Check sheet for the modelled part. Datum: model origin and axes. Units: mm. A direction names the side the tool comes from. Give positions to 0.01 mm unless a question says otherwise; leave off trailing zeros. Write each loop counter-clockwise with the first axis right and the second up, starting at its lowest first coordinate (ties: lowest second). Pieces come first, ordered by that corner, then holes.
from build123d import *
from OCP.BRepFilletAPI import BRepFilletAPI_MakeChamfer

# Parameters (mm, degrees)
SKETCH1_W           = 20.32
SKETCH1_H           = 40.64
BOSS_EXTRUDE1_DEPTH = 25.4
SKETCH2_W           = 20.32
SKETCH2_H           = 40.64
BOSS_EXTRUDE2_DEPTH = 2.38
SKETCH3_W           = 20.32
SKETCH3_H           = 40.5892
BOSS_EXTRUDE3_DEPTH = 4.445
BOSS_EXTRUDE4_DEPTH = 2.38
SKETCH6_R           = 7.62
BOSS_EXTRUDE5_DEPTH = 3.495
CHAMFER1_SIZE       = 2.54
CHAMFER1_SIZE2      = 1.466469684
BOSS_EXTRUDE6_DEPTH = 0.635
SKETCH9_R           = 2.78
BOSS_EXTRUDE7_DEPTH = 7
CHAMFER2_SIZE       = 2.54
CHAMFER2_SIZE2      = 1.466469684
FILLET1_R           = 1
FILLET2_R           = 1.5
SKETCH10_W          = 6.35
SKETCH10_H          = 2.54
SKETCH10_W_2        = 5.08
SKETCH10_H_2        = 1.27
BOSS_EXTRUDE8_DEPTH = 2.4


with BuildPart() as part:
    # Sketch1 → Boss-Extrude1 (new body)
    with BuildSketch(Plane(origin=(0, 0, 0), x_dir=(1, 0, 0), z_dir=(0, 1, 0))):
        with Locations((0, -10.16)):
            Rectangle(SKETCH1_W, SKETCH1_H)
    extrude(amount=BOSS_EXTRUDE1_DEPTH)

    # Sketch2 → Boss-Extrude2 (add)
    with BuildSketch(Plane(origin=(0, 25.4, 0), x_dir=(1, 0, 0), z_dir=(0, 1, 0))):
        with BuildLine():
            ThreePointArc((-5.58, 15.384213562), (-5.08, 12.47), (-4.58, 15.384213562))
            Line((-4.58, 15.384213562), (-4.58, 16.4846))
            Line((-4.58, 16.4846), (4.58, 16.4846))
            Line((4.58, 16.4846), (4.58, 15.384213562))
            ThreePointArc((4.58, 15.384213562), (5.08, 12.47), (5.58, 15.384213562))
            Line((5.58, 15.384213562), (5.58, 16.4846))
            Line((5.58, 16.4846), (10.16, 16.4846))
            Line((10.16, 16.4846), (10.16, 10.16))
            Line((10.16, 10.16), (-10.16, 10.16))
            Line((-10.16, 10.16), (-10.16, 16.4846))
            Line((-10.16, 16.4846), (-5.58, 16.4846))
            Line((-5.58, 16.4846), (-5.58, 15.384213562))
        make_face()
        with Locations((0, -10.16)):
            Rectangle(SKETCH2_W, SKETCH2_H)
        with BuildLine():
            ThreePointArc((5.58, -35.704213562), (5.08, -32.79), (4.58, -35.704213562))
            Line((4.58, -35.704213562), (4.58, -36.8046))
            Line((4.58, -36.8046), (-4.58, -36.8046))
            Line((-4.58, -36.8046), (-4.58, -35.704213562))
            ThreePointArc((-4.58, -35.704213562), (-5.08, -32.79), (-5.58, -35.704213562))
            Line((-5.58, -35.704213562), (-5.58, -36.8046))
            Line((-5.58, -36.8046), (-10.16, -36.8046))
            Line((-10.16, -36.8046), (-10.16, -30.48))
            Line((-10.16, -30.48), (10.16, -30.48))
            Line((10.16, -30.48), (10.16, -36.8046))
            Line((10.16, -36.8046), (5.58, -36.8046))
            Line((5.58, -36.8046), (5.58, -35.704213562))
        make_face()
    extrude(amount=BOSS_EXTRUDE2_DEPTH)

    # Sketch3 → Boss-Extrude3 (add)
    with BuildSketch(Plane(origin=(0, 27.78, 0), x_dir=(1, 0, 0), z_dir=(0, 1, 0))):
        with Locations((0, -10.16)):
            Rectangle(SKETCH3_W, SKETCH3_H)
    extrude(amount=BOSS_EXTRUDE3_DEPTH)

    # Sketch4 → Boss-Extrude4 (add)
    with BuildSketch(Plane(origin=(0, 32.225, 0), x_dir=(1, 0, 0), z_dir=(0, 1, 0))):
        with BuildLine():
            Line((9.652, -18.116559046), (9.652, 3.7846))
            Line((9.652, 3.7846), (4.655896906, 3.7846))
            ThreePointArc((4.655896906, 3.7846), (0, 6.8326), (-4.655896906, 3.7846))
            Line((-4.655896906, 3.7846), (-9.652, 3.7846))
            Line((-9.652, 3.7846), (-9.652, -18.116559046))
            ThreePointArc((-9.652, -18.116559046), (0, -30.2514), (9.652, -18.116559046))
        make_face()
    extrude(amount=BOSS_EXTRUDE4_DEPTH)

    # Sketch6 → Boss-Extrude5 (add)
    with BuildSketch(Plane(origin=(0, 34.605, 0), x_dir=(1, 0, 0), z_dir=(0, 1, 0))):
        with Locations(Location((0, -20.3454, 0), (0, 0, 270))):
            Circle(SKETCH6_R)
    extrude(amount=BOSS_EXTRUDE5_DEPTH)

    # Chamfer1
    chamfer1_edges = [part.edges().sort_by_distance(p)[0] for p in [
        (0, 38.1, 12.7254),
    ]]
    chamfer1_side = [part.faces().sort_by_distance(p)[0] for p in [
        (0, 38.1, 20.3454),
    ]]
    chamfer(chamfer1_edges, length=CHAMFER1_SIZE, length2=CHAMFER1_SIZE2, reference=chamfer1_side[0])

    # Sketch8 → Boss-Extrude6 (add, symmetric)
    with BuildSketch(Plane(origin=(0, 0, 0), x_dir=(0, 0, -1), z_dir=(1, 0, 0))):
        Polygon((-30.4546, 27.78), (-30.4546, 29.48), (-33.2546, 29.48), (-35.7546, 27.78), align=None)
    boss_extrude6 = extrude(amount=BOSS_EXTRUDE6_DEPTH, both=True)

    # Mirror1: Boss-Extrude6 across plane
    add(boss_extrude6.mirror(Plane.XY.offset(10.16)))

    # Sketch9 → Boss-Extrude7 (add)
    with BuildSketch(Plane(origin=(0, 38.1, 0), x_dir=(1, 0, 0), z_dir=(0, 1, 0))):
        with Locations(Location((0, -20.3454, 0), (0, 0, 270))):
            Circle(SKETCH9_R)
    extrude(amount=BOSS_EXTRUDE7_DEPTH)

    # Chamfer2: one chamfer whose edges measure the first distance from different faces: ONE call of the kernel's chamfer builder (chamfer() names one face for all edges)
    chamfer2_edges_1 = [part.edges().sort_by_distance(p)[0] for p in [
        (0, 0, -10.16),
    ]]
    chamfer2_side_1 = [part.faces().sort_by_distance(p)[0] for p in [
        (0, 12.7, -10.16),
    ]]
    chamfer2_edges_2 = [part.edges().sort_by_distance(p)[0] for p in [
        (0, 0, 30.48),
    ]]
    chamfer2_side_2 = [part.faces().sort_by_distance(p)[0] for p in [
        (0, 12.7, 30.48),
    ]]
    chamfer2 = BRepFilletAPI_MakeChamfer(part.part.solid().wrapped)
    for e in chamfer2_edges_1:
        chamfer2.Add(CHAMFER2_SIZE, CHAMFER2_SIZE2, e.wrapped, chamfer2_side_1[0].wrapped)  # the first distance lies on this face
    for e in chamfer2_edges_2:
        chamfer2.Add(CHAMFER2_SIZE, CHAMFER2_SIZE2, e.wrapped, chamfer2_side_2[0].wrapped)  # the first distance lies on this face
    add(Compound.cast(chamfer2.Shape()), mode=Mode.REPLACE)

    # Fillet1
    fillet1_edges = [part.edges().sort_by_distance(p)[0] for p in [
        (-10.16, 30.0025, -10.1346),
        (-10.16, 13.97, -10.16),
        (-10.16, 1.27, -9.426765158),
        (-10.16, 0, 10.16),
        (0, 0, -8.693530316),
        (0, 2.54, -10.16),
        (10.16, 1.27, -9.426765158),
        (10.16, 0, 10.16),
        (0, 0, 29.013530316),
        (10.16, 1.27, 29.746765158),
        (0, 2.54, 30.48),
        (10.16, 13.97, -10.16),
        (10.16, 30.0025, -10.1346),
        (-10.16, 30.0025, 30.4546),
        (10.16, 30.0025, 30.4546),
        (-10.16, 13.97, 30.48),
        (10.16, 13.97, 30.48),
        (-10.16, 1.27, 29.746765158),
    ]]
    fillet(fillet1_edges, radius=FILLET1_R)

    # Fillet2
    fillet2_edges = [part.edges().sort_by_distance(p)[0] for p in [
        (-10.16, 26.59, -16.4846),
        (10.16, 26.59, -16.4846),
        (10.16, 26.59, 36.8046),
        (-10.16, 26.59, 36.8046),
    ]]
    fillet(fillet2_edges, radius=FILLET2_R)

    # Sketch10 → Boss-Extrude8 (add)
    with BuildSketch(Plane(origin=(0, 0, -10.16), x_dir=(-1, 0, 0), z_dir=(0, 0, -1))):
        with Locations((0, 4.32)):
            Rectangle(SKETCH10_W, SKETCH10_H)
        with Locations((0, 4.32)):
            Rectangle(SKETCH10_W_2, SKETCH10_H_2, mode=Mode.SUBTRACT)
    extrude(amount=BOSS_EXTRUDE8_DEPTH)


with BuildPart() as part_1:
    # Body-Move/Copy1: read off the stored shape, not the designer's step
    # Body-Move/Copy1: moved
    add(part.part.moved(Location((0, -40.6, -20.3454))))


solid = part_1.part
1) Sectioned sample at D-D on z = 0. Record the boundary of the cut face in (x, y) (3 decimals).
2) Scan lines: L1, parallel to Z at x = 7, y = -24; L2, parallel to Y at x = 5.5, z = -11.5 (3 decimals); L3, parallel to Z at x = -5.08, y = -14.55. Record each from-to range of solid material in increasing order.
3) Draft check along X on faces 5 (the cylindrical face through (2.289, -4.995, 7.268)), 6 (the flat face through (-9.652, -7, -13)), 7 (the flat face through (-4.58, -14, -36)). Enter one of: +X half, -X half, draft (parallel to the pull), parting line (faces both ways), or undercut.
4) Sectioned sample at A-A on y = -33. Record the boundary of the cut face in (x, z), then the cut area to 3 significant figures.
5) Gauge pin test, flat ends, axial feed: pin 1 (1.4 mm diameter, centred on y = -12, z = -33, fed in from +X) (3 decimals); pin 2 (5.5 mm diameter, centred on x = -2, y = -27, fed in from +Z); pin 3 (3.5 mm diameter, centred on x = 3.5, y = -10, fed in from -Z); pin 4 (2.5 mm diameter, centred on x = -5.08, z = 13.94, fed in from +Y). Record the tip position at first contact, or that the pin passes through.
6) Sectioned sample at B-B on z = -21. Record the boundary of the cut face in (x, y) (3 decimals).
7) Access from +Z, -Z, +X, -X, +Y, -Y to the whole of each face (thin tool, end or side, straight path). Record for faces 1 (the flat face through (7, -7, -24.13)), 2 (the flat face through (0, -35.645, -32)), 3 (the flat face through (0, -35.01, -32)), 4 (the flat face through (-4.58, -14, 16)).
8) Sectioned sample at C-C on y = -9.5. Record the boundary of the cut face in (x, z).
Answers below:
1. outline: (-10.16, -39.6) arc R1 ccw to (-9.16, -40.6) - (9.16, -40.6) arc R1 ccw to (10.16, -39.6) - (10.16, -8.375) - (9.906, -8.375) - (9.906, -5.995) - (7.62, -5.995) - (7.62, -3.966) - (5.08, -2.5) - (2.78, -2.5) - (2.78, 4.5) - (-2.78, 4.5) - (-2.78, -2.5) - (-5.08, -2.5) - (-7.62, -3.966) - (-7.62, -5.995) - (-9.906, -5.995) - (-9.906, -8.375) - (-10.16, -8.375) - close
2. L1: z = -30.51 to 10.13
2. L2: y = -40.6 to -5.995
2. L3: z = -32.82 to 12.44
3. face 5: parting line
3. face 6: -X half
3. face 7: undercut
4. outline: (-10.16, -29.51) arc R1 ccw to (-9.16, -30.51) - (9.16, -30.51) arc R1 ccw to (10.16, -29.51) - (10.16, 9.13) arc R1 ccw to (9.16, 10.13) - (-9.16, 10.13) arc R1 ccw to (-10.16, 9.13) - close
4. area: 825 mm2
5. pin 1: stops at x = 0.635
5. pin 2: stops at z = 10.13
5. pin 3: stops at z = -30.48
5. pin 4: passes through
6. outline: (-10.16, -39.6) arc R1 ccw to (-9.16, -40.6) - (9.16, -40.6) arc R1 ccw to (10.16, -39.6) - (10.16, -8.375) - (9.652, -8.375) - (9.652, -5.995) - (-9.652, -5.995) - (-9.652, -8.375) - (-10.16, -8.375) - close
7. face 1: -Z, +X, +Y
7. face 2: -Z
7. face 3: -Z, +X, -X
7. face 4: +Z, +Y, -Y
8. outline: (-10.16, -29.48) arc R1 ccw to (-9.16, -30.48) - (9.16, -30.48) arc R1 ccw to (10.16, -29.48) - (10.16, 9.11) arc R1 ccw to (9.16, 10.11) - (-9.16, 10.11) arc R1 ccw to (-10.16, 9.11) - close
